from build123d import *

# Parameters (mm, degrees)
SKETCH_1_W          = 2.5
SKETCH_1_H          = 103
SKETCH_1_W_2        = 2
SKETCH_1_H_2        = 95
EXTRUDE_1_DEPTH     = 63
SKETCH_5_W          = 50
SKETCH_5_H          = 2
EXTRUDE_2_DEPTH     = 11
EXTRUDE_3_DEPTH     = 3
CUT_EXTRUDE_1_DEPTH = 4.5
SKETCH_11_W         = 8.5
SKETCH_11_H         = 11.5
CUT_EXTRUDE_2_DEPTH = 4.5
SKETCH_12_W         = 26
SKETCH_12_H         = 28
SKETCH_12_W_2       = 25
SKETCH_12_H_2       = 27
SKETCH_12_W_3       = 8.5
SKETCH_12_H_3       = 11.5
CUT_EXTRUDE_3_DEPTH = 1
SKETCH_13_W         = 30
SKETCH_13_H         = 2
EXTRUDE_4_DEPTH     = 4
EXTRUDE_5_DEPTH     = 3


with BuildPart() as part:
    # 스케치1 → 보스-돌출1 (new body)
    with BuildSketch(Plane(origin=(0, 0, 0), x_dir=(1, 0, 0), z_dir=(0, 1, 0))):
        with Locations((-1, 0)):
            Rectangle(SKETCH_1_W, SKETCH_1_H)
        with Locations((1.25, 0)):
            Rectangle(SKETCH_1_W_2, SKETCH_1_H_2)
    extrude(amount=EXTRUDE_1_DEPTH)

    # 스케치5 → 보스-돌출2 (add)
    with BuildSketch(Plane.ZY.offset(2.25)):
        with Locations((0, 1)):
            Rectangle(SKETCH_5_W, SKETCH_5_H)
    extrude(amount=EXTRUDE_2_DEPTH)

    # 스케치7 → 보스-돌출3 (add)
    with BuildSketch(Plane(origin=(0, 2, 0), x_dir=(1, 0, 0), z_dir=(0, 1, 0))):
        Polygon((-2.25, 23), (-11.25, 23), (-11.25, -23), (-2.25, -23), (-2.25, -25), (-13.25, -25), (-13.25, 25), (-2.25, 25), align=None)
    extrude(amount=EXTRUDE_3_DEPTH)

    # 스케치10 → 컷-돌출1 (cut)
    with BuildSketch(Plane(origin=(2.25, 0, 0), x_dir=(0, 0, -1), z_dir=(1, 0, 0))):
        with BuildLine():
            Line((-20.78, 15.25), (-20.78, 12.25))
            ThreePointArc((-20.78, 12.25), (-12.34, 3.81), (-3.9, 12.25))
            Line((-3.9, 12.25), (-3.9, 15.25))
            ThreePointArc((-3.9, 15.25), (-12.34, 23.69), (-20.78, 15.25))
        make_face()
        with BuildLine():
            Line((4.72, 15.25), (4.72, 12.25))
            ThreePointArc((4.72, 12.25), (13.16, 3.81), (21.6, 12.25))
            Line((21.6, 12.25), (21.6, 15.25))
            ThreePointArc((21.6, 15.25), (13.16, 23.69), (4.72, 15.25))
        make_face()
    extrude(amount=-CUT_EXTRUDE_1_DEPTH, mode=Mode.SUBTRACT)

    # 스케치11 → 컷-돌출2 (cut)
    with BuildSketch(Plane.ZY.offset(2.25)):
        with Locations((0, 46.05)):
            Rectangle(SKETCH_11_W, SKETCH_11_H)
    extrude(amount=-CUT_EXTRUDE_2_DEPTH, mode=Mode.SUBTRACT)

    # 스케치12 → 컷-돌출3 (cut)
    # profile 1 of 2: a face of its own
    with BuildSketch(Plane.ZY.offset(2.25)):
        with Locations((0, 43.5)):
            Rectangle(SKETCH_12_W, SKETCH_12_H)
        with Locations((0, 43.5)):
            Rectangle(SKETCH_12_W_2, SKETCH_12_H_2, mode=Mode.SUBTRACT)
    # profile 2 of 2: a face of its own
    with BuildSketch(Plane.ZY.offset(2.25)):
        with Locations((0, 43.5)):
            Rectangle(SKETCH_12_W_2, SKETCH_12_H_2)
        with Locations((0, 46.05)):
            Rectangle(SKETCH_12_W_3, SKETCH_12_H_3, mode=Mode.SUBTRACT)
    extrude(amount=-CUT_EXTRUDE_3_DEPTH, mode=Mode.SUBTRACT)

    # 스케치13 → 보스-돌출4 (add)
    with BuildSketch(Plane.ZY.offset(2.25)):
        with Locations((0, 28.5)):
            Rectangle(SKETCH_13_W, SKETCH_13_H)
    extrude(amount=EXTRUDE_4_DEPTH)

    # 스케치14 → 보스-돌출5 (add)
    with BuildSketch(Plane(origin=(0, 29.5, 0), x_dir=(1, 0, 0), z_dir=(0, 1, 0))):
        Polygon((-2.25, -13), (-2.25, -15), (-6.25, -15), (-6.25, 15), (-2.25, 15), (-2.25, 13), (-4.25, 13), (-4.25, -13), align=None)
    extrude(amount=EXTRUDE_5_DEPTH)


solid = part.part
The model under review builds one solid part; all positions refer to its coordinate system, in mm. A direction names the side the tool comes from. Round coordinates to 2 decimals unless told otherwise and drop trailing zeros. Loops run counter-clockwise (first coordinate to the right, second up) from the corner with the lowest first, then second, coordinate; pieces in that order, holes last. Notation, with made-up numbers: (-18.75, -0.75) -> (11.25, -0.75) arc R12 ccw to (11.25, 18.25) -> close; hole circle Ø7 at (50, 80). An arc over 180 degrees is marked (long way). One line per question, with ' | ' between items. Start each with the question number.
Item 1: Machinability: for faces 4 (the face through (-4, 30, -15)), 5 (the face through (0, 46, 4.25)), 6 (the face through (-4, 30, 15)), 7 (the face through (-11.25, 3, 0)), 8 (the face through (-8, 2, -25)), which of the approach directions +Z, -Z, +X, -X, +Y, -Y give a long, thin tool a straight path to every point of the face, cutting with its end or side? Answer none if there is none.
Item 2: Draft analysis for pull direction Y (two halves, no side actions). For faces 1 (the face through (0, 40.3, 0)), 2 (the face through (-5, 32.5, 0)), 3 (the face through (-4, 0, -1)), state which applies: +Y half, -Y half, draft (parallel to the pull), parting line (faces both ways), or undercut.
Item 3: Add section A-A, the plane z = -1. Write out the cut boundary in (x, y).
Item 4: Wall thickness on line 1 along Z through (x, y) = (1, 14.5); line 2 along Y through (x, z) = (-10, -12.5); line 3 along X through (y, z) = (35, -21): over which ranges is each line inside the solid? List them lowest first. Write a range as [from, to].
Item 5: Add section C-C, the plane y = 8.5. Write out the cut boundary in (x, z), then the cut area to 3 significant figures.
Item 6: Add section B-B, the plane y = 48. Write out the cut boundary in (x, z).
Item 7: For pin 1 (1.2 mm diameter, centred on x = -5, z = -2.5, fed in from +Y); pin 2 (4 mm diameter, centred on x = -11, z = 7, fed in from +Y); pin 3 (5.5 mm diameter, centred on x = -9.5, y = 1.5, fed in from +Z); pin 4 (0.9 mm diameter, centred on x = -3, y = 44.5, fed in from -Z), all flat-tipped, find the tip position at first contact; note any pin that passes through.
Item 8: Add section D-D, the plane x = -10.25. Write out the cut boundary in (y, z), then the cut area to 3 significant figures.
Return value:
1) face 4: -Z, -X, +Y | face 5: +X, -X | face 6: +Z, -X, +Y | face 7: +Y | face 8: -Z, -X, +Y, -Y
2) face 1: undercut | face 2: +Y half | face 3: -Y half
3) outline: (-13.25, 0) -> (2.25, 0) -> (2.25, 40.3) -> (-1.25, 40.3) -> (-1.25, 29.5) -> (-4.25, 29.5) -> (-4.25, 32.5) -> (-6.25, 32.5) -> (-6.25, 27.5) -> (-2.25, 27.5) -> (-2.25, 2) -> (-11.25, 2) -> (-11.25, 5) -> (-13.25, 5) -> close; (-2.25, 57.5) -> (-1.25, 57.5) -> (-1.25, 51.8) -> (2.25, 51.8) -> (2.25, 63) -> (-2.25, 63) -> close
4) line 1: z = [-47.5, -21.6], [-4.72, 3.9], [20.78, 47.5] | line 2: y = [0, 2] | line 3: x = [-2.25, 2.25]
5) outline: (-2.25, -51.5) -> (0.25, -51.5) -> (0.25, -47.5) -> (2.25, -47.5) -> (2.25, -20.72) -> (-2.25, -20.72) -> close; (-2.25, -5.6) -> (2.25, -5.6) -> (2.25, 4.78) -> (-2.25, 4.78) -> close; (-2.25, 19.9) -> (2.25, 19.9) -> (2.25, 47.5) -> (0.25, 47.5) -> (0.25, 51.5) -> (-2.25, 51.5) -> close | area: 311 mm2
6) outline: (-2.25, -51.5) -> (0.25, -51.5) -> (0.25, -47.5) -> (2.25, -47.5) -> (2.25, -4.25) -> (-1.25, -4.25) -> (-1.25, -13) -> (-2.25, -13) -> close; (-2.25, 13) -> (-1.25, 13) -> (-1.25, 4.25) -> (2.25, 4.25) -> (2.25, 47.5) -> (0.25, 47.5) -> (0.25, 51.5) -> (-2.25, 51.5) -> close
7) pin 1: stops at y = 32.5 | pin 2: stops at y = 5 | pin 3: stops at z = 25 | pin 4: passes through
8) outline: (0, -25) -> (5, -25) -> (5, -23) -> (2, -23) -> (2, 23) -> (5, 23) -> (5, 25) -> (0, 25) -> close | area: 112 mm2
